Job drawing, mm, ordinate dimensions from the low corner. One solid piece. Coordinates: 2 decimals unless noted, no trailing zeros. Loops run counter-clockwise (first coordinate to the right, second up) from the corner with the lowest first, then second, coordinate; pieces in that order, holes last. Notation, with made-up numbers: (-29, -11) - (20, -11) arc R15 cw to (20, 4) - close; hole circle Ø10 at (54.25, 12.5). An arc over 180 degrees is marked (long way). Use a Markdown table: item, result. Add a question column.
1) Drop flat-ended pins along their axis: P1, Ø4, axis at y = 7.51, z = 6.5, coming from the -X side; P2, Ø1, axis at x = 1, y = 2, coming from the -Z side; P3, Ø1.5, axis at y = 9, z = 9, coming from the +X side. Give the stop position or say it passes through.
2) Probe probe 1 along Z at (x, y) = (0.75, 6.5); probe 2 along Y at (x, z) = (2.5, 4.25) (1 decimal); probe 3 along Z at (x, y) = (4.75, 10). List the from-to ranges inside material, lowest first. Write a range as [from, to].
3) Pull direction Z, two halves, no side cores. Call the marked faces 1, 2 and 3: +Z half, -Z half, draft (parallel to the pull), parting line (faces both ways), or undercut.
4) Band-saw the part on A-A (x = 4.75). Give the cut face in (y, z) (1 decimal).
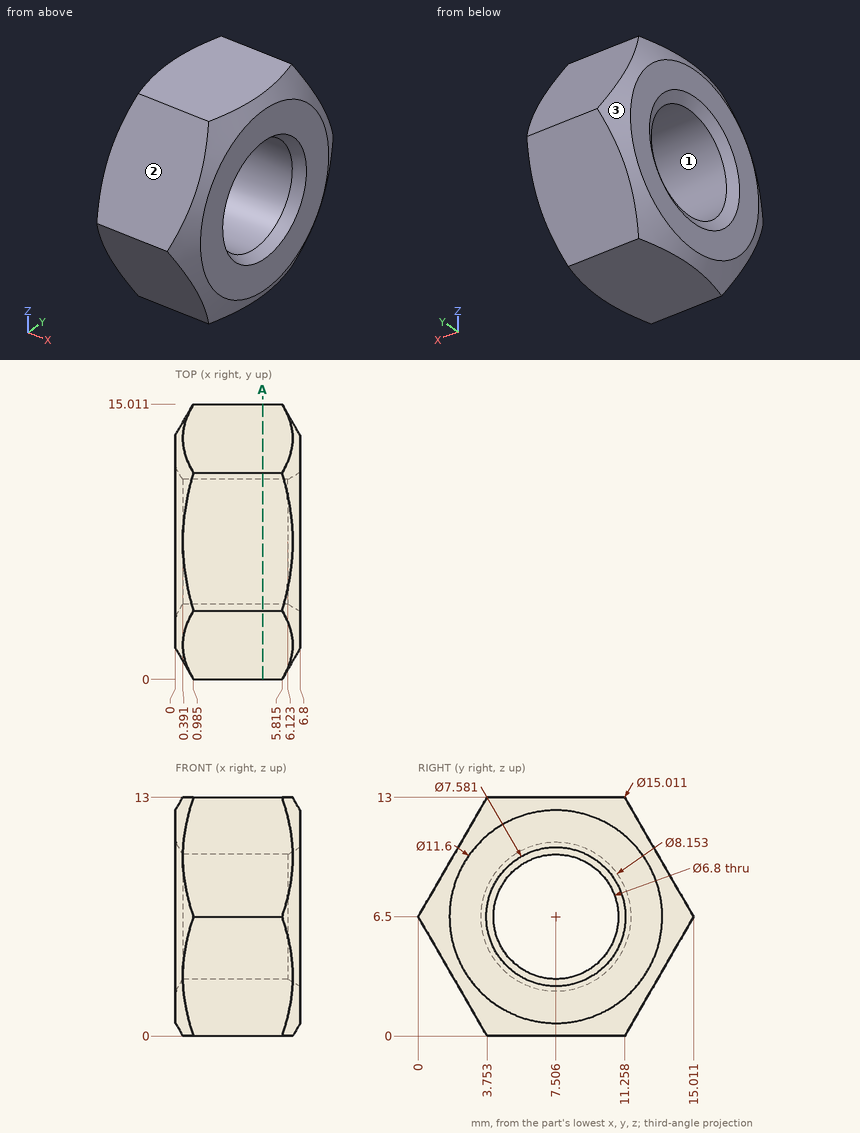
Answer block:
| question | item | result |
|---|---|---|
| 1 | P1 | through |
| 1 | P2 | z = 2.17 |
| 1 | P3 | x = 6.58 |
| 2 | probe 1 | [0, 3.25], [9.75, 13] |
| 2 | probe 2 | [1.3, 5], [10.1, 13.7] |
| 2 | probe 3 | [0, 4.19], [8.81, 13] |
| 3 | face 1 | undercut |
| 3 | face 2 | +Z half |
| 3 | face 3 | parting line |
| 4 | outline | (0, 6.5) - (3.8, 0) - (11.3, 0) - (15, 6.5) - (11.3, 13) - (3.8, 13) - close; hole circle Ø6.8 at (7.5, 6.5) |
